Input: part model. Units: mm. Frame: model coordinates. A direction names the side the tool comes from. Round coordinates to 2 decimals unless told otherwise and drop trailing zeros. Loops run counter-clockwise (first coordinate to the right, second up) from the corner with the lowest first, then second, coordinate; pieces in that order, holes last. Notation, with made-up numbers: (2, 50.5) - (32, 50.5) arc R15 ccw to (32, 78.5) - close; hole circle Ø9 at (-38, 14.5). An arc over 180 degrees is marked (long way). Use CSV: the item, a comma, the result in double quotes. Start each with the question number.
1. Material intervals for probe 1 along Z at (x, y) = (-39, 328.5); probe 2 along X at (y, z) = (112, -92); probe 3 along X at (y, z) = (200, -35), sorted ascending. Write a range as from..to.
2. Cut plane D-D (y = 520). Return loops of the section in (x, z), and give its area (3 significant figures).
3. Cut plane C-C (x = -31.5). Return loops of the section in (y, z).
4. Cut plane B-B (z = 50). Return loops of the section in (x, y), and give its area (3 significant figures).
5. Pull-direction query (X, two-part tool) for faces 1 (the flat face through (-6, 78, 39.624)), 2 (the flat face through (94.488, 131, 69)), 3 (the flat face through (45.11, 100.18, -87.02)), 4 (the flat face through (197, 0, -87)); classes: +X half, -X half, draft (parallel to the pull), parting line (faces both ways), or undercut.
6. Access query for faces 5 (the flat face through (-82.956, 100.178, -63.398)), 6 (the flat face through (73, 131, -112.776)), 7 (the flat face through (-8, 78, -61.976)), 8 (the flat face through (116, 79, -61.976)). Directions: +Z, -Z, +X, -X, +Y, -Y. A direction counts if a zero-diameter tool reaches every point of the face in a straight line with its end or side. Return the directions, or none.
7. Cut plane A-A (y = 86). Return loops of the section in (x, z), and give its area (3 significant figures).
8. Pin query (flat end, axial travel): P1, Ø4, axis at y = 101, z = 74, coming from the -X side; P2, Ø12, axis at y = 240, z = 80, coming from the -X side. Return the tip coordinate at first contact, or that it passes through.
```python
from build123d import *

# Parameters (mm, degrees)
SKETCH1_W           = 101.6
SKETCH1_H           = 101.6
BOSS_EXTRUDE1_DEPTH = 812.8
BOSS_EXTRUDE2_DEPTH = 50.8
BOSS_EXTRUDE3_DEPTH = 50.8
BOSS_EXTRUDE4_DEPTH = 50.8
BOSS_EXTRUDE6_DEPTH = 50.8


with BuildPart() as part:
    # Sketch1 → Boss-Extrude1 (new body)
    with BuildSketch(Plane(origin=(0, 0, 0), x_dir=(1, 0, 0), z_dir=(0, 1, 0))):
        with Locations((-7.112, 11.176)):
            Rectangle(SKETCH1_W, SKETCH1_H)
    extrude(amount=BOSS_EXTRUDE1_DEPTH)

    # Sketch2 → Boss-Extrude2 (add)
    with BuildSketch(Plane.ZY.offset(57.912)):
        Polygon((-163.576, 0), (39.624, 203.2), (39.624, 304.8), (-265.176, 0), align=None)
    extrude(amount=BOSS_EXTRUDE2_DEPTH)

    # Sketch3 → Boss-Extrude3 (add)
    with BuildSketch(Plane(origin=(0, 0, -61.976), x_dir=(-1, 0, 0), z_dir=(0, 0, -1))):
        Polygon((-145.288, 0), (57.912, 203.2), (57.912, 304.8), (-246.888, 0), align=None)
    extrude(amount=BOSS_EXTRUDE3_DEPTH)

    # Sketch5 → Boss-Extrude4 (add)
    with BuildSketch(Plane.XY.offset(39.624)):
        Polygon((-159.512, 0), (43.688, 203.2), (43.688, 304.8), (-261.112, 0), align=None)
    extrude(amount=BOSS_EXTRUDE4_DEPTH)

    # Sketch7 → Boss-Extrude6 (add)
    with BuildSketch(Plane(origin=(43.688, 0, 0), x_dir=(0, 0, -1), z_dir=(1, 0, 0))):
        Polygon((-141.224, 0), (61.976, 203.2), (61.976, 304.8), (-242.824, 0), align=None)
    extrude(amount=BOSS_EXTRUDE6_DEPTH)


solid = part.part
```
Established:
1,probe 1,"z = -61.98..39.62"
1,probe 2,"x = -108.71..-57.91, 33.29..134.89"
1,probe 3,"x = -108.71..94.49"
2,outline,"(-57.91, -61.98) - (43.69, -61.98) - (43.69, 39.62) - (-57.91, 39.62) - close"
2,area,"10,300 mm2"
3,outline,"(0, -61.98) - (176.79, -61.98) - (176.79, -112.78) - (278.39, -112.78) - (278.39, -61.98) - (812.8, -61.98) - (812.8, 39.62) - (229.61, 39.62) - (229.61, 90.42) - (128.01, 90.42) - (128.01, 39.62) - (0, 39.62) - close"
4,outline,"(-261.11, 0) - (-159.51, 0) - (43.69, 203.2) - (43.69, 304.8) - close; (43.69, 91.22) - (94.49, 91.22) - (94.49, 192.82) - (43.69, 192.82) - close"
4,area,"31,000 mm2"
5,face 1,"undercut"
5,face 2,"+X half"
5,face 3,"undercut"
5,face 4,"draft"
6,face 5,"-X, -Y"
6,face 6,"-Z, +X, +Y, -Y"
6,face 7,"-Z, -Y"
6,face 8,"+X, -Y"
7,outline,"(-175.11, 39.62) - (-73.51, 39.62) - (-73.51, 90.42) - (-175.11, 90.42) - close; (-108.71, -179.18) - (-57.91, -179.18) - (-57.91, -77.58) - (-108.71, -77.58) - close; (-57.91, -61.98) - (43.69, -61.98) - (43.69, 39.62) - (-57.91, 39.62) - close; (43.69, 55.22) - (94.49, 55.22) - (94.49, 156.82) - (43.69, 156.82) - close; (59.29, -112.78) - (160.89, -112.78) - (160.89, -61.98) - (59.29, -61.98) - close"
7,area,"31,000 mm2"
8,P1,"stops at x = -162.11"
8,P2,"stops at x = -27.11"
